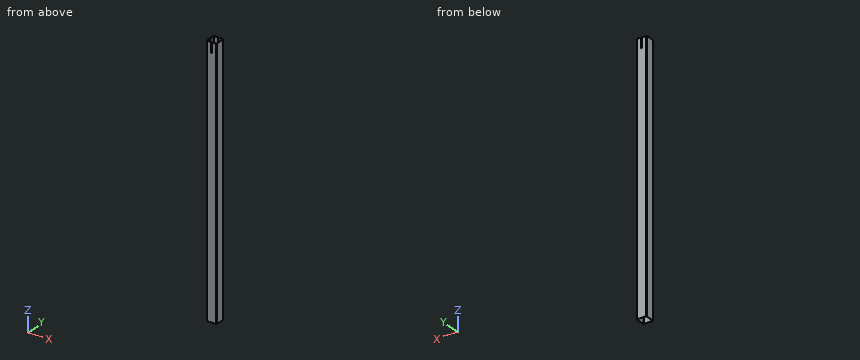
```python
from build123d import *

# Parameters (mm, degrees)
EXTRUDE_1_DEPTH     = 2600
CUT_EXTRUDE_1_DEPTH = 100


with BuildPart() as part:
    # Эскиз1 → Бобышка-Вытянуть1 (new body)
    with BuildSketch(Plane.XY):
        with BuildLine():
            Line((-44, 50), (44, 50))
            ThreePointArc((44, 50), (48.242640687, 48.242640687), (50, 44))
            Line((50, 44), (50, -44))
            ThreePointArc((50, -44), (48.242640687, -48.242640687), (44, -50))
            Line((44, -50), (-44, -50))
            ThreePointArc((-44, -50), (-48.242640687, -48.242640687), (-50, -44))
            Line((-50, -44), (-50, 44))
            ThreePointArc((-50, 44), (-48.242640687, 48.242640687), (-44, 50))
        make_face()
        with BuildLine():
            Line((-43, 47), (43, 47))
            ThreePointArc((43, 47), (45.828427125, 45.828427125), (47, 43))
            Line((47, 43), (47, -43))
            ThreePointArc((47, -43), (45.828427125, -45.828427125), (43, -47))
            Line((43, -47), (-43, -47))
            ThreePointArc((-43, -47), (-45.828427125, -45.828427125), (-47, -43))
            Line((-47, -43), (-47, 43))
            ThreePointArc((-47, 43), (-45.828427125, 45.828427125), (-43, 47))
        make_face(mode=Mode.SUBTRACT)
    extrude(amount=-EXTRUDE_1_DEPTH)

    # Эскиз2 → Вырез-Вытянуть1 (cut)
    with BuildSketch(Plane.XY):
        Polygon((-50, 3), (-3, 3), (-3, 50), (3, 50), (3, 3), (50, 3), (50, -3), (3, -3), (3, -50), (-3, -50), (-3, -3), (-50, -3), align=None)
    extrude(amount=-CUT_EXTRUDE_1_DEPTH, mode=Mode.SUBTRACT)


solid = part.part
```
Can you work these out from the model? Positions are in its coordinate system, mm. Give positions to 0.01 mm unless a question says otherwise; leave off trailing zeros. Loops run counter-clockwise (first coordinate to the right, second up) from the corner with the lowest first, then second, coordinate; pieces in that order, holes last. Notation, with made-up numbers: M 86,19 L 125,19 A27 cw 125,52 Z; hole C 26,14.5 d1. An arc over 180 degrees is marked long. Use one line per item in the form item = value. Start each with the question number.
(1) Please list where this line runs through material, in increasing order: line 1 (Y direction, x = -18, z = -1241).
(2) I want a section at A-A, the plane x = 22. Write out the boundary of the cut face in (y, z), and give its area (3 significant figures).
(3) I'm going to push flat-ended pins straight in: P1, Ø2.5, axis at y = 48, z = -71.5, coming from the -X side; P2, Ø2.5, axis at x = 1, y = 48, coming from the +Z side; P3, Ø2.5, axis at x = -48.5, z = -28, coming from the -Y side. Where does each tip first touch, or does it pass through?
(4) I want a section at C-C, the plane z = -1509.5. Write out the boundary of the cut face in (x, y).
Worked out:
q1.line_1 = -50 to -47, 47 to 50
q2.outline = M -50,-2600 L -47,-2600 L -47,0 L -50,0 Z; M 47,-2600 L 50,-2600 L 50,0 L 47,0 Z
q2.area = 15,600 mm²
q3.P1 = -49.33
q3.P2 = -100
q3.P3 = -49.04
q4.outline = M -50,-44 A6 ccw -44,-50 L 44,-50 A6 ccw 50,-44 L 50,44 A6 ccw 44,50 L -44,50 A6 ccw -50,44 Z; hole M -47,-43 A4 ccw -43,-47 L 43,-47 A4 ccw 47,-43 L 47,43 A4 ccw 43,47 L -43,47 A4 ccw -47,43 Z
